from build123d import *

# Parameters (mm, degrees)
BOSS_EXTRUDE1_DEPTH     = 0.5953125
CIRPATTERN1_COUNT       = 4
SKETCH6_W               = 30
SKETCH6_H               = 30
BOSS_EXTRUDE2_DEPTH     = 20
CUT_EXTRUDE2_DEPTH      = 25.636
CUT_EXTRUDE2_DEPTH_BACK = 0.254
SKETCH8_W               = 27.7
SKETCH8_H               = 27.7


with BuildPart() as part:
    # Sketch1 → Revolve2 (revolve)
    with BuildSketch(Plane.XY):
        Polygon((0, 0), (0, 152.4), (12.7, 125.16476211), (12.7, 6.35), (10.80240754, 6.35), (8.89, 0), align=None)
    revolve(axis=Axis((0, -1000, 0), (0, 1, 0)))

    # Sketch3 → Boss-Extrude1 (add, symmetric)
    with BuildSketch(Plane.XY):
        Polygon((11.1125, 66.023452099), (28.575, 28.575), (28.575, -4.7625), (11.1125, 12.7), align=None)
    boss_extrude1 = extrude(amount=BOSS_EXTRUDE1_DEPTH, both=True)

    # CirPattern1: Boss-Extrude1 ×4 about axis
    cirpattern1_axis = Axis((0, 0, 0), (0, 1, 0))
    for i in range(1, CIRPATTERN1_COUNT):
        add(boss_extrude1.rotate(cirpattern1_axis, i * 360 / CIRPATTERN1_COUNT))

    # Sketch5 → Cut-Revolve1 (revolve, cut)
    with BuildSketch(Plane.XY):
        Polygon((8.061034129, 0), (0, 0), (0, 95.25), (11.1125, 95.25), (11.1125, 10.132154301), align=None)
    revolve(axis=Axis((0, -1000, 0), (0, 1, 0)), mode=Mode.SUBTRACT)

    # Sketch6 → Boss-Extrude2 (add)
    with BuildSketch(Plane(origin=(-5.901898503, 3.807192265, 0), x_dir=(1, 0, 0), z_dir=(0, 0, 1))):
        with Locations((5.85297619, 92.047729896)):
            Rectangle(SKETCH6_W, SKETCH6_H)
    extrude(amount=BOSS_EXTRUDE2_DEPTH)

    # Sketch8 → Cut-Extrude2 (cut, two sides: drawn at the far end of the back side and taken through both)
    with BuildSketch(Plane(origin=(72.442949274, -2.579929792, 0), x_dir=(1, 0, 0), z_dir=(0, 0, 1)).offset(-CUT_EXTRUDE2_DEPTH_BACK)):
        with Locations((-72.46037851, 98.457547314)):
            Rectangle(SKETCH8_W, SKETCH8_H)
    extrude(amount=CUT_EXTRUDE2_DEPTH + CUT_EXTRUDE2_DEPTH_BACK, mode=Mode.SUBTRACT)


solid = part.part
Input: part model. Units: mm. Frame: model coordinates. A direction names the side the tool comes from. Coordinates: 2 decimals unless noted, no trailing zeros. Loops run counter-clockwise (first coordinate to the right, second up) from the corner with the lowest first, then second, coordinate; pieces in that order, holes last. Notation, with made-up numbers: (19, 51.25) -> (78, 51.25) arc R27 ccw to (78, 83.25) -> close; hole circle Ø5 at (51, -26). An arc over 180 degrees is marked (long way). One line per item, written item: value.
(1) Cut plane D-D (x = -18). Output: boundary loops of the cut face in (y, z), then the cut area to 3 significant figures.
Answer below:
outline: (5.81, -0.6) -> (51.25, -0.6) -> (51.25, 0.6) -> (5.81, 0.6) -> close
area: 54.1 mm2
(2) Ray query, line 1 along Y through (x, z) = (7, 6.5); line 2 along Z through (x, y) = (0, 75); line 3 along X through (y, z) = (12, 20.5). Return the intervals inside material, ascending.
Answer below:
line 1: y = 2.2 to 4.95, 80.85 to 82.03, 109.73 to 131.91
line 2: z = -12.7 to -11.11, 11.11 to 12.7
line 3: x = -0.6 to 0.6
(3) Cut plane C-C (y = 68.5). Output: boundary loops of the cut face in (x, z) (1 decimal), then the cut area to 3 significant figures.
Answer below:
outline: circle Ø25.4 at (0, 0); hole circle Ø22.2 at (0, 0)
area: 119 mm2
(4) Cut plane B-B (z = 24.5). Output: boundary loops of the cut face in (x, y), then the cut area to 3 significant figures.
Answer below:
outline: (-0.6, -0.69) -> (0.6, -0.69) -> (0.6, 37.31) -> (-0.6, 37.31) -> close
area: 45.2 mm2
(5) Pin query (flat end, axial travel): pin 1 Ø12.5 at (x, y) = (-17, 16.5) entering from +Z; pin 2 Ø6 at (y, z) = (97, 9.5) entering from -X; pin 3 Ø12.5 at (x, y) = (17, 27) entering from -Z. Return the tip coordinate at first contact, or that it passes through.
Answer below:
pin 1: stops at z = 6.76
pin 2: stops at x = -15.05
pin 3: stops at z = -6.76
(6) Draft query along X for faces 4 (the face through (-21, 29, 0.595)), 5 (the face through (20.74, 3.07, 0.01)), 6 (the face through (-15.049, 96, 10)). Return one class per face: pulls with the +X half, pulls with the -X half, needs draft (parallel to the pull), parting line crosses it, or undercut.
Answer below:
face 4: needs draft
face 5: undercut
face 6: pulls with the -X half
(7) Cut plane A-A (y = 13.5). Output: boundary loops of the cut face in (x, z) (1 decimal).
Answer below:
outline: (-28.6, -0.6) -> (-12.7, -0.6) arc R12.7 ccw to (-0.6, -12.7) -> (-0.6, -28.6) -> (0.6, -28.6) -> (0.6, -12.7) arc R12.7 ccw to (12.7, -0.6) -> (28.6, -0.6) -> (28.6, 0.6) -> (12.7, 0.6) arc R12.7 ccw to (0.6, 12.7) -> (0.6, 28.6) -> (-0.6, 28.6) -> (-0.6, 12.7) arc R12.7 ccw to (-12.7, 0.6) -> (-28.6, 0.6) -> close; hole circle Ø22.2 at (0, 0)
(8) Set-up query: faces 1 (the face through (-13.867, 96, 10)), 2 (the face through (0, 102, -0.254)), 3 (the face through (-21, 29, -0.595)). Return all of +Z, -Z, +X, -X, +Y, -Y with unobstructed straight access to the full face (end or side cutting, diameter ignored); none if empty.
Answer below:
face 1: +Z, -Z
face 2: +Z, +X, -X
face 3: -Z, -X, +Y, -Y
